```python
from build123d import *

# Parameters (mm, degrees)
SKETCH1_R           = 1.25
BOSS_EXTRUDE1_DEPTH = 2
FILLET1_R           = 2.5


with BuildPart() as part:
    # Sketch1 → Boss-Extrude1 (new body)
    with BuildSketch(Plane(origin=(0, 0, 0), x_dir=(1, 0, 0), z_dir=(0, 1, 0))):
        with BuildLine():
            Line((-103.965757813, 67.162425071), (-33.817700106, 107.662425071))
            Line((-33.817700106, 107.662425071), (-14.010882201, 73.356010123))
            ThreePointArc((-14.010882201, 73.356010123), (-9.775048525, 74.210673935), (-8.39729226, 70.115002459))
            Line((-8.39729226, 70.115002459), (31.216343551, 70.115002459))
            Line((31.216343551, 70.115002459), (31.216343551, -10.884997541))
            Line((31.216343551, -10.884997541), (-8.39729226, -10.884997541))
            ThreePointArc((-8.39729226, -10.884997541), (-9.775048525, -14.980669016), (-14.010882201, -14.126005204))
            Line((-14.010882201, -14.126005204), (-33.817700106, -48.432420153))
            Line((-33.817700106, -48.432420153), (-103.965757813, -7.932420153))
            Line((-103.965757813, -7.932420153), (-84.158939907, 26.373994796))
            ThreePointArc((-84.158939907, 26.373994796), (-87.017017318, 29.615002459), (-84.158939907, 32.856010123))
            Line((-84.158939907, 32.856010123), (-103.965757813, 67.162425071))
        make_face()
        with Locations(Location((-83.75035682, 29.615002459, 0), (0, 0, 270))):
            Circle(SKETCH1_R, mode=Mode.SUBTRACT)
        with Locations(Location((-11.408378774, 71.381662958, 0), (0, 0, 270))):
            Circle(SKETCH1_R, mode=Mode.SUBTRACT)
        with Locations(Location((-11.408378774, -12.151658039, 0), (0, 0, 270))):
            Circle(SKETCH1_R, mode=Mode.SUBTRACT)
        Polygon((-76.69928593, 29.615002459), (-14.933914219, 65.275256443), (-14.933914219, -6.045251524), align=None, mode=Mode.SUBTRACT)
    extrude(amount=BOSS_EXTRUDE1_DEPTH)

    # Fillet1
    fillet1_edges = [part.edges().sort_by_distance(p)[0] for p in [
        (-14.010882201, 1, -73.356010123),
        (-8.39729226, 1, -70.115002459),
        (-8.39729226, 1, 10.884997541),
        (-14.010882201, 1, 14.126005204),
        (-84.158939907, 1, -26.373994796),
        (-84.158939907, 1, -32.856010123),
        (-14.933914219, 1, -65.275256443),
        (-76.69928593, 1, -29.615002459),
        (-14.933914219, 1, 6.045251524),
    ]]
    fillet(fillet1_edges, radius=FILLET1_R)


solid = part.part
```
Verification items for the finished model (mm, model axes). A direction names the side the tool comes from. Coordinates: 2 decimals unless noted, no trailing zeros. Write each loop counter-clockwise with the first axis right and the second up, starting at its lowest first coordinate (ties: lowest second). Pieces come first, ordered by that corner, then holes. Notation, with made-up numbers: M -2.75,64.25 L 42.25,64.25 A16 cw 42.25,84.25 Z; hole C 32.25,43.5 d4. An arc over 180 degrees is marked long. Answer as a JSON object with one key per item and string values. Group by question number.
(1) Cross-section at C-C, the plane y = 0.65. Record the cut outline in (x, z) (3 decimals), and give its area (3 significant figures).
(2) Material ranges on line 1 (X direction, y = 1.4, z = -37); line 2 (Z direction, x = -29.5, y = 0.75); line 3 (X direction, y = 1.1, z = -4.5), recorded low to high.
(3) Gauge pin test, flat ends, axial feed: pin 1 (0.6 mm diameter, centred on x = 17, y = 1.5, fed in from +Z) (3 decimals); pin 2 (2 mm diameter, centred on x = -11.41, z = 12.15, fed in from +Y); pin 3 (0.6 mm diameter, centred on x = 10.5, y = 1, fed in from -Z) (3 decimals). Record the tip position at first contact, or that the pin passes through.
(4) Cross-section at B-B, the plane x = -17. Record the cut outline in (y, z).
(5) Tool access check on faces 1 (the face through (-69.38, 0.99, -87.13)), 2 (the face through (-94.59, 0.99, -50.92)), 3 (the face through (-45.437, 0.986, -11.566)). Record the directions out of +Z, -Z, +X, -X, +Y, -Y that give a thin tool (end or side, any length) a straight path to the whole face; none if there is none.
(6) Cross-section at A-A, the plane z = -47.5. Record the cut outline in (x, y).
(7) Cross-section at D-D, the plane z = 34.5. Record the cut outline in (x, y).
(8) Release check for a two-part mould opening along X. For faces 4 (the face through (-94.85, 0.99, -7.86)), 5 (the face through (-24.7, 0.99, -91.87)), 6 (the face through (-46.196, 0.986, -47.226)) record: +X half, -X half, draft (parallel to the pull), parting line (faces both ways), or undercut.
Reply:
{
 "1": {"outline": "M -103.966,-67.162 L -33.818,-107.662 L -15.322,-75.627 A2.5 cw -12.399,-74.495 A3.267 ccw -8.217,-72.08 A2.5 cw -5.775,-70.115 L 31.216,-70.115 L 31.216,10.885 L -5.775,10.885 A2.5 cw -8.217,12.85 A3.267 ccw -12.399,15.265 A2.5 cw -15.322,16.397 L -33.818,48.432 L -103.966,7.932 L -85.47,-24.103 A2.5 cw -85.951,-27.201 A3.267 ccw -85.951,-32.029 A2.5 cw -85.47,-35.127 Z; hole C -83.75,-29.615 d2.5; hole M -72.949,-31.78 L -18.684,-63.11 A2.5 ccw -14.934,-60.945 L -14.934,1.715 A2.5 ccw -18.684,3.88 L -72.949,-27.45 A2.5 ccw Z; hole C -11.408,-71.382 d2.5; hole C -11.408,12.152 d2.5", "area": "11,200 mm²"},
 "2": {"line 1": "-86.55 to -63.91, -14.93 to 31.22", "line 2": "-100.18 to -56.87, -2.36 to 40.95", "line 3": "-96.79 to -33.2, -14.93 to 31.22"},
 "3": {"pin 1": "z = 10.885", "pin 2": "through", "pin 3": "z = -70.115"},
 "4": {"outline": "M 0,-78.53 L 2,-78.53 L 2,-63.41 L 0,-63.41 Z; M 0,4.18 L 2,4.18 L 2,19.3 L 0,19.3 Z"},
 "5": {"face 1": "-Z, -X, +Y, -Y", "face 2": "-X, +Y, -Y", "face 3": "+Y, -Y"},
 "6": {"outline": "M -92.61,0 L -45.72,0 L -45.72,2 L -92.61,2 Z; M -14.93,0 L 31.22,0 L 31.22,2 L -14.93,2 Z"},
 "7": {"outline": "M -57.95,0 L -25.77,0 L -25.77,2 L -57.95,2 Z"},
 "8": {"face 4": "-X half", "face 5": "+X half", "face 6": "undercut"}
}
